CAD build for the part. Positions are in the model's coordinates, mm. A direction names the side the tool comes from. Round coordinates to 2 decimals unless told otherwise and drop trailing zeros. Order: outer loops, then holes, each group sorted by start corner. A loop starts at its lowest first (then second) coordinate and runs counter-clockwise, first axis right, second up. Notation, with made-up numbers: M -5,-6.75 L 16,-6.75 A18 ccw 16,6.25 Z; hole C 11,18 d4. An arc over 180 degrees is marked long. Answer as a JSON object with one key per item and string values.
```python
from build123d import *

# Parameters (mm, degrees)
SKETCH1_R                                      = 12.5
SKETCH1_R_2                                    = 7.14375
BOSS_EXTRUDE1_DEPTH                            = 10
SKETCH2_R                                      = 12.5
BOSS_EXTRUDE2_DEPTH                            = 1.5
CHAMFER1_SIZE                                  = 3.75
CHAMFER1_SIZE2                                 = 6.495190528
SKETCH8_R                                      = 7.75
SKETCH8_R_2                                    = 3.05
BOSS_EXTRUDE3_DEPTH                            = 2.5
CSK_FOR_M2_FLAT_HEAD_MACHINE_SCREW1_AT_2_COUNT = 2
CSK_FOR_M2_FLAT_HEAD_MACHINE_SCREW1_AT_2_PITCH = 5
SKETCH16_R                                     = 0.75
CUT_EXTRUDE1_DEPTH                             = 22.089096709
M2X0_4_TAPPED_HOLE1_D                          = 1.6
M2X0_4_TAPPED_HOLE1_CSINK_D                    = 2.4
M2X0_4_TAPPED_HOLE1_CSINK_ANGLE                = 90
CUT_EXTRUDE2_DEPTH                             = 2.5
FILLET1_R                                      = 1


with BuildPart() as part:
    # Sketch1 → Boss-Extrude1 (new body)
    with BuildSketch(Plane(origin=(0, 0, 0), x_dir=(1, 0, 0), z_dir=(0, 1, 0))):
        with Locations(Location((0, 0, 0), (0, 0, 270))):
            Circle(SKETCH1_R)
        with Locations(Location((0, 0, 0), (0, 0, 270))):
            Circle(SKETCH1_R_2, mode=Mode.SUBTRACT)
    extrude(amount=BOSS_EXTRUDE1_DEPTH)

    # Sketch2 → Boss-Extrude2 (add)
    with BuildSketch(Plane(origin=(0, 10, 0), x_dir=(1, 0, 0), z_dir=(0, 1, 0))):
        with Locations(Location((0, 0, 0), (0, 0, 270))):
            Circle(SKETCH2_R)
    extrude(amount=BOSS_EXTRUDE2_DEPTH)

    # Chamfer1
    chamfer1_edges = [part.edges().sort_by_distance(p)[0] for p in [
        (0, 0, -12.5),
    ]]
    chamfer1_side = [part.faces().sort_by_distance(p)[0] for p in [
        (0, 0, -12.146446609),
    ]]
    chamfer(chamfer1_edges, length=CHAMFER1_SIZE, length2=CHAMFER1_SIZE2, reference=chamfer1_side[0])

    # Sketch8 → Boss-Extrude3 (add)
    with BuildSketch(Plane(origin=(0, 11.5, 0), x_dir=(1, 0, 0), z_dir=(0, 1, 0))):
        with Locations(Location((0, 0, 0), (0, 0, 270))):
            Circle(SKETCH8_R)
        with Locations(Location((0, 0, 0), (0, 0, 270))):
            Circle(SKETCH8_R_2, mode=Mode.SUBTRACT)
    extrude(amount=BOSS_EXTRUDE3_DEPTH)

    # Sketch11 → CSK for M2 Flat Head Machine Screw1 (revolve, cut)
    with BuildSketch(Plane(origin=(-1.767766953, 11.5, 1.767766953), x_dir=(0, 0, 1), z_dir=(1, 0, 0))):
        Polygon((0, 0), (0, 11.5), (1.2, 11.5), (1.2, 1), (2.2, 0), align=None)
    csk_for_m2_flat_head_machine_screw1 = revolve(axis=Axis((-1.767766953, 17.85, 1.767766953), (0, -1, 0)), mode=Mode.SUBTRACT)

    # CSK for M2 Flat Head Machine Screw1 at 2: CSK for M2 Flat Head Machine Screw1 ×2
    with Locations(*[Vector(0.707106781186547, 0, -0.707106781186548) * (i * CSK_FOR_M2_FLAT_HEAD_MACHINE_SCREW1_AT_2_PITCH) for i in range(1, CSK_FOR_M2_FLAT_HEAD_MACHINE_SCREW1_AT_2_COUNT)]):
        add(csk_for_m2_flat_head_machine_screw1, mode=Mode.SUBTRACT)

    # Sketch16 → Cut-Extrude1 (cut, through all)
    with BuildSketch(Plane(origin=(0, 11.5, 0), x_dir=(1, 0, 0), z_dir=(0, 1, 0))):
        with Locations(Location((0, 0, 0), (0, 0, 270))):
            Circle(SKETCH16_R)
    extrude(amount=-CUT_EXTRUDE1_DEPTH, mode=Mode.SUBTRACT)

    # M2x0.4 Tapped Hole1 (through all)
    with Locations(Plane(origin=(3.181980515, 14, 3.181980515), x_dir=(0, 0, 1), z_dir=(0, 1, 0))):
        with Locations((0, 0), (-6.36396103, -6.36396103)):
            CounterSinkHole(M2X0_4_TAPPED_HOLE1_D / 2, M2X0_4_TAPPED_HOLE1_CSINK_D / 2, counter_sink_angle=M2X0_4_TAPPED_HOLE1_CSINK_ANGLE)

    # Sketch20 → Cut-Extrude2 (cut)
    with BuildSketch(Plane(origin=(0, 14, 0), x_dir=(1, 0, 0), z_dir=(0, 1, 0))):
        with BuildLine():
            ThreePointArc((0.019981986, -3.049934544), (0.42751991, -1.911696068), (0.172083929, -0.729991179))
            ThreePointArc((0.172083929, -0.729991179), (-0.530330086, -0.530330086), (-0.729991179, 0.172083929))
            ThreePointArc((-0.729991179, 0.172083929), (-1.911696068, 0.42751991), (-3.049934544, 0.019981986))
            ThreePointArc((-3.049934544, 0.019981986), (-3.323401872, -3.323401872), (0.019981986, -3.049934544))
        make_face()
        with BuildLine():
            ThreePointArc((-0.019981986, 3.049934544), (-0.42751991, 1.911696068), (-0.172083929, 0.729991179))
            ThreePointArc((-0.172083929, 0.729991179), (0.530330086, 0.530330086), (0.729991179, -0.172083929))
            ThreePointArc((0.729991179, -0.172083929), (1.911696068, -0.42751991), (3.049934544, -0.019981986))
            ThreePointArc((3.049934544, -0.019981986), (3.323401872, 3.323401872), (-0.019981986, 3.049934544))
        make_face()
    extrude(amount=-CUT_EXTRUDE2_DEPTH, mode=Mode.SUBTRACT)

    # Fillet1
    fillet1_edges = [part.edges().sort_by_distance(p)[0] for p in [
        (0, 11.5, -12.5),
        (0, 11.5, -7.75),
    ]]
    fillet(fillet1_edges, radius=FILLET1_R)


solid = part.part
```
Item 1: Saw through at B-B on y = 5.75. List the corners of the cut face in (x, z), and give its area (3 significant figures).
Worked answers:
{"outline": "C 0,0 d24.14; hole C 0,0 d14.29", "area": "297 mm2"}
Item 2: Drop flat-ended pins along their axis: pin 1 Ø3.5 at (x, z) = (1.77, -1.77) entering from +Y; pin 2 Ø1 at (y, z) = (6.5, 3.5) entering from -X; pin 3 Ø1.8 at (x, z) = (-3.18, -3.18) entering from +Y. Give the stop position or say it passes through.
Worked answers:
{"pin 1": "stops at y = 11.05", "pin 2": "stops at x = -12.13", "pin 3": "stops at y = 13.7"}
Item 3: 3-axis set-ups, long thin cutter, end or side, ignore diameter. For faces 1 (the cylindrical face through (-3.361, 12.768, 3.285)), 2 (the cylindrical face through (-0.665, 10.761, 0.346)), 3 (the flat face through (-1, 10, 0)): which of +Z, -Z, +X, -X, +Y, -Y reach the whole face in a straight line?
Worked answers:
{"face 1": "+Y", "face 2": "+Y, -Y", "face 3": "-Y"}
Item 4: Saw through at A-A on y = 3.25. List the corners of the cut face in (x, z).
Worked answers:
{"outline": "C 0,0 d21.25; hole C 0,0 d14.29"}
Item 5: Two-plate mould, pull along Z, no slides. Class faces 4 (the flat face through (-3.3, 14, -0.1)), 5 (the cylindrical face through (3.755, 8.47, 11.923)), 6 (the cylindrical face through (3.975, 11.775, 3.286)): released by +Z, released by -Z, zero draft, split by the parting line, or undercut.
Worked answers:
{"face 4": "zero draft", "face 5": "split by the parting line", "face 6": "undercut"}
Item 6: Wall check: line 1 along X through (y, z) = (9, -3); line 2 along Z through (x, y) = (5.25, 2.25); line 3 along Z through (x, y) = (5.25, 4.5). Give the ranges that are in metal, low to high. Write a range as [from, to].
Worked answers:
{"line 1": "x = [-12.13, -6.48], [6.48, 12.13]", "line 2": "z = [-8.57, -4.84], [4.84, 8.57]", "line 3": "z = [-10.06, -4.84], [4.84, 10.06]"}
